Work out the finished part from the listing and answer in its coordinate system (mm). Face numbers are marked on the shaded views. A direction names the side the tool comes from. Coordinates: 2 decimals unless noted, no trailing zeros. Write each loop counter-clockwise with the first axis right and the second up, starting at its lowest first coordinate (ties: lowest second). Pieces come first, ordered by that corner, then holes. Notation, with made-up numbers: M 3,-38 L 18,-38 A18 ccw 18,-15 Z; hole C -31.75,-18 d1. An arc over 180 degrees is marked long. Answer as CSV lines item,"result". Start each with the question number.
(1) For the marked faces 1, 2, 3, 4 and 5, determine the directions among +Z, -Z, +X, -X, +Y, -Y from which every point of the face is accessible in a straight line to the end or side of a thin tool.
(2) A cutting plane is placed at C-C on z = 15. Give the vertices of the cut face in (x, y), then the cut area to 4 significant figures.
(3) A cutting plane is placed at B-B on y = 85.5. Give the vertices of the cut face in (x, z), then the cut area to 3 significant figures.
(4) Find the intervals of material crossed by L1, parallel to Z at x = 61, y = 86; L2, parallel to Y at x = 59, z = 11.5; L3, parallel to Z at x = 59, y = 82, in increasing order. Write a range as [from, to].
(5) A cutting plane is placed at A-A on x = 56.75. Give the vertices of the cut face in (y, z), then the cut area to 3 significant figures.
(6) A cutting plane is placed at D-D on y = 72. Give the vertices of the cut face in (x, z).
(7) Flat-ended cylindrical pins translate along their axes: P1, Ø3, axis at x = 53, y = 63, coming from the -Z side; P2, Ø5, axis at x = 60, z = 3.5, coming from the -Y side; P3, Ø3, axis at x = 57.54, y = 85.89, coming from the +Z side; P4, Ø6, axis at x = 56.5, y = 87, coming from the -Z side. Find the tip coordinate at first contact, or state that the pin passes through.
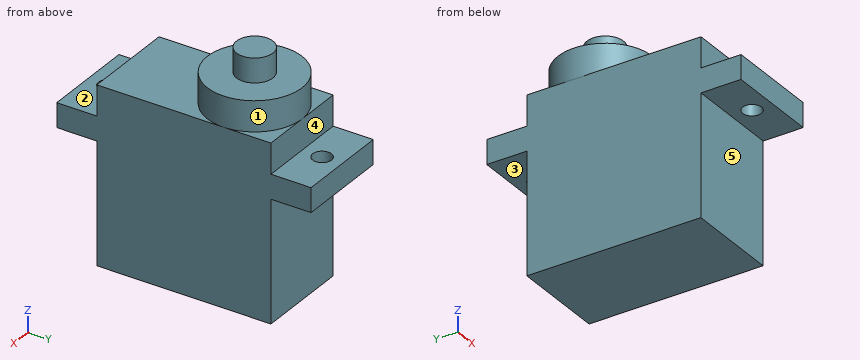
Solid Edge part; units mm, degrees
sketch "Sketch1" plane through (0, 0, 0) normal (0, 0, 1) x (1, 0, 0)
  line L0 (51.2908, 60.2391) -> (63.7908, 60.2391)
  line L1 (63.7908, 60.2391) -> (63.7908, 83.2391)
  line L2 (63.7908, 83.2391) -> (51.2908, 83.2391)
  line L3 (51.2908, 83.2391) -> (51.2908, 60.2391)
extrude "Protrusion1" add sketch "Sketch1" along normal blind 16
sketch "Sketch2" plane through (57.5408, 71.7391, 16) normal (0, 0, 1) x (1, 0, 0)
  circle A0 centre (0, 14.15) radius 1.25
  circle A1 centre (0, -14.15) radius 1.25
  line L0 (-6.25, 16.8) -> (6.25, 16.8)
  line L1 (6.25, 16.8) -> (6.25, -16.8)
  line L2 (6.25, -16.8) -> (-6.25, -16.8)
  line L3 (-6.25, -16.8) -> (-6.25, 16.8)
extrude "flange" add sketch "Sketch2" along normal blind 3.2
sketch "Sketch3" plane through (57.5408, 71.7391, 19.2) normal (0, 0, 1) x (1, 0, 0)
  line L0 (-6.25, 11.5) -> (6.25, 11.5)
  line L1 (6.25, 11.5) -> (6.25, -11.5)
  line L2 (6.25, -11.5) -> (-6.25, -11.5)
  line L3 (-6.25, -11.5) -> (-6.25, 11.5)
extrude "top" add sketch "Sketch3" along normal blind 4
sketch "Sketch4" plane through (57.5408, 71.7391, 23.2) normal (0, 0, 1) x (1, 0, 0)
  circle A0 centre (0, 5.25) radius 6.25
extrude "ExtrudedProtrusion_4" add sketch "Sketch4" along normal blind 4
sketch "Sketch5" plane through (57.5408, 76.9891, 27.2) normal (0, 0, 1) x (0, 1, 0)
  circle A0 centre (0, 0) radius 2.4
extrude "ExtrudedProtrusion_5" add sketch "Sketch5" along normal blind 3.2
Here are the results:
1,face 1,"+Z"
1,face 2,"+Z, +X, -X, -Y"
1,face 3,"-Z, +X, -X, +Y"
1,face 4,"+Z, +X, -X, +Y"
1,face 5,"-Z, +X, -X, -Y"
2,outline,"M 51.29,60.24 L 63.79,60.24 L 63.79,83.24 L 51.29,83.24 Z"
2,area,"287.5 mm^2"
3,outline,"M 51.29,16 L 56.35,16 L 56.35,19.2 L 51.29,19.2 Z; M 58.73,16 L 63.79,16 L 63.79,19.2 L 58.73,19.2 Z"
3,area,"32.4 mm^2"
4,L1,"z = [16, 19.2]"
4,L2,"y = [60.24, 83.24]"
4,L3,"z = [0, 27.2]"
5,outline,"M 54.94,16 L 56.62,16 L 56.62,19.2 L 54.94,19.2 Z; M 58.56,16 L 60.24,16 L 60.24,0 L 83.24,0 L 83.24,16 L 84.92,16 L 84.92,19.2 L 83.24,19.2 L 83.24,23.2 L 83.19,23.2 L 83.19,27.2 L 79.26,27.2 L 79.26,30.4 L 74.72,30.4 L 74.72,27.2 L 70.79,27.2 L 70.79,23.2 L 60.24,23.2 L 60.24,19.2 L 58.56,19.2 Z; M 86.86,16 L 88.54,16 L 88.54,19.2 L 86.86,19.2 Z"
5,area,"619 mm^2"
6,outline,"M 51.29,0 L 63.79,0 L 63.79,23.2 L 61.31,23.2 L 61.31,27.2 L 53.78,27.2 L 53.78,23.2 L 51.29,23.2 Z"
7,P1,"stops at z = 0"
7,P2,"stops at y = 60.24"
7,P3,"stops at z = 19.2"
7,P4,"stops at z = 16"
